Here's how the part is built. I have some questions about the finished solid (model axes, mm). Face numbers are marked on the shaded views. Coordinates: 2 decimals unless noted, no trailing zeros. Write each loop counter-clockwise with the first axis right and the second up, starting at its lowest first coordinate (ties: lowest second). Pieces come first, ordered by that corner, then holes.
(1) Imagine slicing it at B-B, the plane y = -31.5. List the corners of the cut face in (x, z) for me.
(2) Imagine slicing it at D-D, the plane y = -64.5. List the corners of the cut face in (x, z) for me, plus the area to 3 significant figures.
(3) Imagine slicing it at A-A, the plane z = 11. List the corners of the cut face in (x, y) for me.
(4) For pin 1 Ø0.5 at (x, z) = (-42.5, 7.5) entering from +Y; pin 2 Ø9 at (x, z) = (-30, 2.5) entering from -Y; pin 3 Ø12 at (x, z) = (50.5, 16.5) entering from -Y; pin 4 Ø9 at (y, z) = (-21.5, 3) entering from -X, each with a flat end and sliding along its axis, tell me the tip position at first contact or that it passes through.
(5) Thinking about a two-plate mould opening in Y: for the marked faces 1 and 2, which applies, released by +Y, released by -Y, zero draft, split by the parting line, or undercut?
(6) Please list where these lines run through material, in increasing order: probe 1 along Y at (x, z) = (131.5, 11.5); probe 2 along X at (y, z) = (74.5, 7); probe 3 along Z at (x, y) = (-120.5, 24).
(7) Imagine slicing it at C-C, the plane x = 91. List the corners of the cut face in (y, z) for me, plus the area to 3 significant figures.
```python
from build123d import *

# Parameters (mm, degrees)
F0_W     = 320
F0_H     = 250
F1_DEPTH = 20
F3_DEPTH = 12
F5_DEPTH = 1.6
F6_W     = 33
F6_H     = 100
F6_W_2   = 150
F6_H_2   = 33
F7_DEPTH = 20.001


with BuildPart() as f1:
    # F0 (on Top) → F1 (new body)
    with BuildSketch(Plane.XY):
        Rectangle(F0_W, F0_H)
    extrude(amount=F1_DEPTH)

    # F2 (on face) → F3 (cut)
    with BuildSketch(Plane.XY.offset(20)):
        with BuildLine():
            ThreePointArc((148.3, 109.5), (145.8, 112), (148.3, 114.5))
            Line((148.3, 114.5), (-148.3, 114.5))
            ThreePointArc((-148.3, 114.5), (-146.532233047, 113.767766953), (-145.8, 112))
            ThreePointArc((-145.8, 112), (-146.532233047, 110.232233047), (-148.3, 109.5))
            Line((-148.3, 109.5), (-148.3, -109.5))
            ThreePointArc((-148.3, -109.5), (-146.532233047, -110.232233047), (-145.8, -112))
            ThreePointArc((-145.8, -112), (-146.532233047, -113.767766953), (-148.3, -114.5))
            Line((-148.3, -114.5), (148.3, -114.5))
            ThreePointArc((148.3, -114.5), (145.8, -112), (148.3, -109.5))
            Line((148.3, -109.5), (148.3, 109.5))
        make_face()
        with BuildLine():
            ThreePointArc((150.8, 112), (150.067766953, 113.767766953), (148.3, 114.5))
            Line((148.3, 114.5), (148.3, 109.5))
            ThreePointArc((148.3, 109.5), (150.067766953, 110.232233047), (150.8, 112))
        make_face()
        with BuildLine():
            Line((148.3, 109.5), (148.3, 114.5))
            ThreePointArc((148.3, 114.5), (145.8, 112), (148.3, 109.5))
        make_face()
        with BuildLine():
            ThreePointArc((-145.8, 112), (-146.532233047, 113.767766953), (-148.3, 114.5))
            Line((-148.3, 114.5), (-148.3, 109.5))
            ThreePointArc((-148.3, 109.5), (-146.532233047, 110.232233047), (-145.8, 112))
        make_face()
        with BuildLine():
            Line((-148.3, 109.5), (-148.3, 114.5))
            ThreePointArc((-148.3, 114.5), (-150.8, 112), (-148.3, 109.5))
        make_face()
        with BuildLine():
            ThreePointArc((150.8, -112), (150.067766953, -110.232233047), (148.3, -109.5))
            Line((148.3, -109.5), (148.3, -114.5))
            ThreePointArc((148.3, -114.5), (150.067766953, -113.767766953), (150.8, -112))
        make_face()
        with BuildLine():
            Line((148.3, -114.5), (148.3, -109.5))
            ThreePointArc((148.3, -109.5), (145.8, -112), (148.3, -114.5))
        make_face()
        with BuildLine():
            ThreePointArc((-145.8, -112), (-146.532233047, -110.232233047), (-148.3, -109.5))
            Line((-148.3, -109.5), (-148.3, -114.5))
            ThreePointArc((-148.3, -114.5), (-146.532233047, -113.767766953), (-145.8, -112))
        make_face()
        with BuildLine():
            Line((-148.3, -114.5), (-148.3, -109.5))
            ThreePointArc((-148.3, -109.5), (-150.8, -112), (-148.3, -114.5))
        make_face()
    extrude(amount=-F3_DEPTH, mode=Mode.SUBTRACT)

    # F4 (on face) → F5 (cut)
    with BuildSketch(Plane.XY.offset(8)):
        with BuildLine():
            ThreePointArc((123.2, 86.8), (121.7, 88.3), (123.2, 89.8))
            Line((123.2, 89.8), (-123.2, 89.8))
            ThreePointArc((-123.2, 89.8), (-122.1393398282, 89.3606601718), (-121.7, 88.3))
            ThreePointArc((-121.7, 88.3), (-122.1393398282, 87.2393398282), (-123.2, 86.8))
            Line((-123.2, 86.8), (-123.2, -86.8))
            ThreePointArc((-123.2, -86.8), (-122.1393398282, -87.2393398282), (-121.7, -88.3))
            ThreePointArc((-121.7, -88.3), (-122.1393398282, -89.3606601718), (-123.2, -89.8))
            Line((-123.2, -89.8), (123.2, -89.8))
            ThreePointArc((123.2, -89.8), (121.7, -88.3), (123.2, -86.8))
            Line((123.2, -86.8), (123.2, 86.8))
        make_face()
        with BuildLine():
            ThreePointArc((124.7, 88.3), (124.2606601718, 89.3606601718), (123.2, 89.8))
            Line((123.2, 89.8), (123.2, 86.8))
            ThreePointArc((123.2, 86.8), (124.2606601718, 87.2393398282), (124.7, 88.3))
        make_face()
        with BuildLine():
            Line((123.2, 86.8), (123.2, 89.8))
            ThreePointArc((123.2, 89.8), (121.7, 88.3), (123.2, 86.8))
        make_face()
        with BuildLine():
            ThreePointArc((-121.7, 88.3), (-122.1393398282, 89.3606601718), (-123.2, 89.8))
            Line((-123.2, 89.8), (-123.2, 86.8))
            ThreePointArc((-123.2, 86.8), (-122.1393398282, 87.2393398282), (-121.7, 88.3))
        make_face()
        with BuildLine():
            Line((-123.2, 86.8), (-123.2, 89.8))
            ThreePointArc((-123.2, 89.8), (-124.7, 88.3), (-123.2, 86.8))
        make_face()
        with BuildLine():
            ThreePointArc((124.7, -88.3), (124.2606601718, -87.2393398282), (123.2, -86.8))
            Line((123.2, -86.8), (123.2, -89.8))
            ThreePointArc((123.2, -89.8), (124.2606601718, -89.3606601718), (124.7, -88.3))
        make_face()
        with BuildLine():
            Line((123.2, -89.8), (123.2, -86.8))
            ThreePointArc((123.2, -86.8), (121.7, -88.3), (123.2, -89.8))
        make_face()
        with BuildLine():
            ThreePointArc((-121.7, -88.3), (-122.1393398282, -87.2393398282), (-123.2, -86.8))
            Line((-123.2, -86.8), (-123.2, -89.8))
            ThreePointArc((-123.2, -89.8), (-122.1393398282, -89.3606601718), (-121.7, -88.3))
        make_face()
        with BuildLine():
            Line((-123.2, -89.8), (-123.2, -86.8))
            ThreePointArc((-123.2, -86.8), (-124.7, -88.3), (-123.2, -89.8))
        make_face()
    extrude(amount=-F5_DEPTH, mode=Mode.SUBTRACT)

    # F6 (on face) → F7 (cut, through all)
    with BuildSketch(Plane.XY.offset(20)):
        with Locations((-160, 0)):
            Rectangle(F6_W, F6_H)
        with Locations((0, 125)):
            Rectangle(F6_W_2, F6_H_2)
        with Locations((160, 0)):
            Rectangle(F6_W, F6_H)
        with Locations((0, -125)):
            Rectangle(F6_W_2, F6_H_2)
    extrude(amount=-F7_DEPTH, mode=Mode.SUBTRACT)


solid = f1.part
```
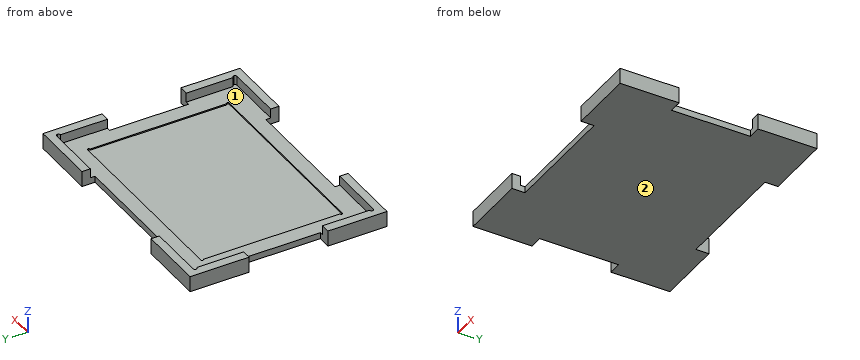
Recorded:
1. outline: (-143.5, 0) - (143.5, 0) - (143.5, 8) - (123.2, 8) - (123.2, 6.4) - (-123.2, 6.4) - (-123.2, 8) - (-143.5, 8) - close
2. outline: (-160, 0) - (160, 0) - (160, 20) - (148.3, 20) - (148.3, 8) - (123.2, 8) - (123.2, 6.4) - (-123.2, 6.4) - (-123.2, 8) - (-148.3, 8) - (-148.3, 20) - (-160, 20) - close
2. area: 2,450 mm2
3. outline: (-160, -125) - (-75, -125) - (-75, -114.5) - (-148.3, -114.5) arc R2.5 cw to (-148.3, -109.5) - (-148.3, -50) - (-160, -50) - close; (-160, 50) - (-148.3, 50) - (-148.3, 109.5) arc R2.5 cw to (-148.3, 114.5) - (-75, 114.5) - (-75, 125) - (-160, 125) - close; (75, -125) - (160, -125) - (160, -50) - (148.3, -50) - (148.3, -109.5) arc R2.5 cw to (148.3, -114.5) - (75, -114.5) - close; (75, 114.5) - (148.3, 114.5) arc R2.5 cw to (148.3, 109.5) - (148.3, 50) - (160, 50) - (160, 125) - (75, 125) - close
4. pin 1: stops at y = 108.5
4. pin 2: stops at y = -108.5
4. pin 3: passes through
4. pin 4: stops at x = -143.5
5. face 1: undercut
5. face 2: zero draft
6. probe 1: y = -125 to -114.5, 114.5 to 125
6. probe 2: x = -160 to -123.2, 123.2 to 160
6. probe 3: z = 0 to 6.4
7. outline: (-125, 0) - (125, 0) - (125, 20) - (114.5, 20) - (114.5, 8) - (89.8, 8) - (89.8, 6.4) - (-89.8, 6.4) - (-89.8, 8) - (-114.5, 8) - (-114.5, 20) - (-125, 20) - close
7. area: 1,960 mm2
